Autodesk Inventor part; units mm, degrees
ref_plane "YZ Plane" through (0, 0, 0) normal (1, 0, 0) x (0, 1, 0)
ref_plane "XZ Plane" through (0, 0, 0) normal (0, 1, 0) x (-1, 0, 0)
ref_plane "XY Plane" through (0, 0, 0) normal (0, 0, 1) x (1, 0, 0)
sketch "Sketch1" plane through (0, 0, 0) normal (0, 0, 1) x (1, 0, 0)
  line L0 (1.5875, 0) -> (106.3625, 0)
  line L1 (107.95, 1.5875) -> (107.95, 55.5625)
  line L2 (106.3625, 57.15) -> (1.5875, 57.15)
  line L3 (0, 55.5625) -> (0, 1.5875)
  arc A0 (1.5875, 57.15) -> (0, 55.5625) centre (1.5875, 55.5625) ccw
  arc A1 (107.95, 55.5625) -> (106.3625, 57.15) centre (106.3625, 55.5625) ccw
  arc A2 (106.3625, 0) -> (107.95, 1.5875) centre (106.3625, 1.5875) ccw
  arc A3 (0, 1.5875) -> (1.5875, 0) centre (1.5875, 1.5875) ccw
  point P0 (0, 0)
  point P1 (107.95, 0)
  point P2 (0, 57.15)
  dimension "d0" = 57.15
  dimension "d1" = 107.95
  dimension "d2" = 1.5875
  dimension "d3" = 1.5875
extrude "Extrusion1" add sketch "Sketch1" along normal blind 6.35
sketch "Sketch2" plane through (0, 0, 6.35) normal (0, 0, 1) x (1, 0, 0)
  line L0 (104.775, 52.3875) -> (104.775, 4.7625)
  line L1 (3.175, 4.7625) -> (3.175, 52.3875)
  arc A0 (4.7625, 53.975) -> (3.175, 52.3875) centre (4.7625, 52.3875) ccw
  arc A1 (104.775, 52.3875) -> (103.1875, 53.975) centre (103.1875, 52.3875) ccw
  arc A2 (103.1875, 3.175) -> (104.775, 4.7625) centre (103.1875, 4.7625) ccw
  arc A3 (3.175, 4.7625) -> (4.7625, 3.175) centre (4.7625, 4.7625) ccw
  line L2 (106.3625, 57.15) -> (1.5875, 57.15)
  line L3 (107.95, 1.5875) -> (107.95, 55.5625)
  line L4 (1.5875, 0) -> (106.3625, 0)
  line L5 (0, 55.5625) -> (0, 1.5875)
  arc A4 (6.35, 53.975) -> (12.7, 53.975) centre (9.525, 53.975) ccw
  arc A5 (95.25, 53.975) -> (101.6, 53.975) centre (98.425, 53.975) ccw
  arc A6 (101.6, 3.175) -> (95.25, 3.175) centre (98.425, 3.175) ccw
  arc A7 (12.7, 3.175) -> (6.35, 3.175) centre (9.525, 3.175) ccw
  line L6 (4.7625, 53.975) -> (6.35, 53.975)
  line L7 (12.7, 53.975) -> (95.25, 53.975)
  line L8 (101.6, 53.975) -> (103.1875, 53.975)
  line L9 (103.1875, 3.175) -> (101.6, 3.175)
  line L10 (95.25, 3.175) -> (12.7, 3.175)
  line L11 (6.35, 3.175) -> (4.7625, 3.175)
  point P0 (0, 0)
  dimension "d6" = 1.5875
  dimension "d8" = 3.175
  dimension "d10" = 3.175
  dimension "d11" = 6.35
  dimension "d12" = 6.35
  dimension "d43" = 3.175
extrude "Extrusion2" cut sketch "Sketch2" against normal blind 3.175
fillet "Fillet1" radius 1.5875 8 edges at (0.465, 56.685, 0) (0, 28.575, 0) (0.465, 0.465, 0) (53.975, 0, 0) (107.485, 0.465, 0) (107.95, 28.575, 0) (107.485, 56.685, 0) (53.975, 57.15, 0)
sketch "Sketch3" plane through (0, 0, 3.175) normal (0, 0, 1) x (1, 0, 0)
  line L0 (28.575, 54.0321) -> (79.375, 54.0321)
  line L1 (79.375, 54.0321) -> (79.375, 50.8571)
  line L2 (79.375, 50.8571) -> (28.575, 50.8571)
  line L3 (28.575, 50.8571) -> (28.575, 54.0321)
  line L4 (3.175, 4.7625) -> (3.175, 52.3875)
  line L5 (3.175, 41.275) -> (6.35, 41.275)
  line L6 (6.35, 41.275) -> (6.35, 15.875)
  line L7 (6.35, 15.875) -> (3.175, 15.875)
  line L8 (3.175, 15.875) -> (3.175, 41.275)
  line L9 (104.775, 52.3875) -> (104.775, 4.7625)
  line L10 (104.775, 41.275) -> (101.6, 41.275)
  line L11 (101.6, 41.275) -> (101.6, 15.875)
  line L12 (101.6, 15.875) -> (104.775, 15.875)
  line L13 (104.775, 15.875) -> (104.775, 41.275)
  line L14 (95.25, 3.175) -> (12.7, 3.175)
  line L15 (79.375, 3.175) -> (28.575, 3.175)
  line L16 (28.575, 3.175) -> (28.575, 5.461)
  line L17 (28.575, 5.461) -> (79.375, 5.461)
  line L18 (79.375, 5.461) -> (79.375, 3.175)
  line L19 (103.1875, 3.175) -> (101.6, 3.175)
  line L20 (101.6, 53.975) -> (103.1875, 53.975)
  point P0 (0, 0)
  point P1 (28.575, 4.318)
  point P2 (79.375, 4.318)
  point P3 (79.375, 52.4446)
  point P4 (4.7625, 41.275)
  point P5 (103.1875, 41.275)
  point P6 (103.1875, 15.875)
  point P7 (4.7625, 15.875)
  point P8 (102.3937, 3.175)
  dimension "d16" = 25.4
  dimension "d17" = 25.4
  dimension "d18" = 2.286
  dimension "d19" = 3.175
  dimension "d20" = 3.175
  dimension "d21" = 3.175
  dimension "d22" = 12.7
  dimension "d23" = 12.7
extrude "Extrusion3" add sketch "Sketch3" along normal blind 6.35
hole "Hole1" at (9.525, 53.975, 6.35) at (98.425, 53.975, 6.35) at (98.425, 3.175, 6.35) at (9.525, 3.175, 6.35) direction (0, 0, -1) diameter 3.175 end through all
sketch "Sketch5" plane through (0, 0, 0) normal (0, 0, -1) x (-1, 0, 0)
  line L0 (-28.702, 18.2245) -> (-19.558, 18.2245)
  line L1 (-19.558, 18.2245) -> (-19.558, 9.0805)
  line L2 (-19.558, 9.0805) -> (-28.702, 9.0805)
  line L3 (-28.702, 9.0805) -> (-28.702, 18.2245)
  line L4 (-1.5875, 1.5875) -> (-106.3625, 1.5875)
  line L5 (-1.5875, 55.5625) -> (-1.5875, 1.5875)
  point P0 (0, 0)
  point P1 (-24.13, 9.0805)
  dimension "d36" = 7.493
  dimension "d37" = 17.9705
  dimension "d38" = 9.144
  dimension "d39" = 9.144
extrude "Extrusion4" cut sketch "Sketch5" against normal blind 6.35
fillet "Fillet2" radius 1.5875 4 edges at (24.13, 18.2245, 0) (19.558, 13.6525, 0) (28.702, 13.6525, 0) (24.13, 9.0805, 0)
sketch "Sketch7" plane through (0, 0, 3.175) normal (0, 0, 1) x (1, 0, 0)
  line L0 (79.375, 7.239) -> (53.975, 7.239)
  line L1 (53.975, 7.239) -> (53.975, 10.414)
  line L2 (53.975, 10.414) -> (79.375, 10.414)
  line L3 (79.375, 10.414) -> (79.375, 7.239)
  line L4 (79.375, 3.175) -> (79.375, 6.35)
  line L5 (28.575, 5.461) -> (79.375, 5.461)
  point P0 (0, 0)
  point P1 (79.375, 5.461)
  dimension "d48" = 3.175
  dimension "d49" = 25.4
  dimension "d50" = 0
  dimension "d51" = 1.778
extrude "Extrusion6" add sketch "Sketch7" along normal blind 6.35
chamfer "Chamfer2" distance 2.286 angle 45 1 edges at (53.975, 5.461, 9.525)
sketch "Sketch8" plane through (0, 0, 0) normal (0, 0, -1) x (-1, 0, 0)
  circle A0 centre (-98.425, 53.975) radius 1.5875
  circle A1 centre (-9.525, 53.975) radius 1.5875
  circle A2 centre (-9.525, 3.175) radius 1.5875
  arc A3 (-95.25, 3.175) -> (-101.6, 3.175) centre (-98.425, 3.175) ccw
  point P0 (0, 0)
  point P1 (-9.525, 1.5875)
hole "Hole2" at (98.425, 53.975, 0) at (9.525, 53.975, 0) at (9.525, 3.175, 0) at (98.425, 3.175, 0) direction (0, 0, 1) diameter 3.175 depth 6.35 tip angle 118 counterbore diameter 5.334 counterbore depth 2.54
properties part number "Case_Rear"
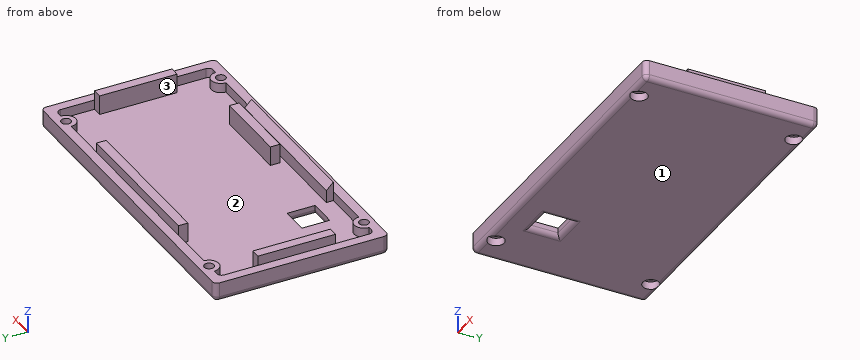
Can you work these out from the model? Positions are in its coordinate system, mm. Face numbers are marked on the shaded views. Coordinates: 2 decimals unless noted, no trailing zeros. Answer as a JSON object with one key per item and string values.
1) For P1, Ø5, axis at x = 9.525, y = 3.175, coming from the -Z side; P2, Ø5, axis at x = 76.5, y = 33.5, coming from the +Z side (3 decimals); P3, Ø1.1, axis at y = 4.5, z = 8, coming from the -X side (3 decimals), each with a flat end and sliding along its axis, tell me the tip position at first contact or that it passes through.
Results:
{"P1": "stops at z = 2.54", "P2": "stops at z = 3.175", "P3": "stops at x = 28.575"}
2) Imagine slicing it at D-D (z = 4.75). Count the separate pieces of the cut face and the enclosed holes in it, then the cut area to 3 significant figures.
Results:
{"separate pieces": "2", "enclosed holes": "5", "area": "1,560 mm^2"}
3) Thinking about a two-plate mould opening in X: for the marked faces 1, 2 and 3, which applies, pulls with the +X half, pulls with the -X half, needs draft (parallel to the pull), parting line crosses it, or undercut?
Results:
{"face 1": "needs draft", "face 2": "undercut", "face 3": "undercut"}
4) If I drill on line 1 (Y direction, x = 59, z = 6.75) (3 decimals); line 2 (Y direction, x = 75.5, z = 4); line 3 (Y direction, x = 52, z = 5.5), over which ranges is the centre line in solid material (lowest first)?
Results:
{"line 1": "y = 3.175 to 5.461, 7.239 to 10.414, 50.857 to 54.032", "line 2": "y = 0 to 5.46, 7.24 to 10.41, 50.86 to 57.15", "line 3": "y = 0 to 5.46, 50.86 to 57.15"}
